Autodesk Inventor part; units mm, degrees
ref_plane "YZ Plane" through (0, 0, 0) normal (1, 0, 0) x (0, 1, 0)
ref_plane "XZ Plane" through (0, 0, 0) normal (0, 1, 0) x (-1, 0, 0)
ref_plane "XY Plane" through (0, 0, 0) normal (0, 0, 1) x (1, 0, 0)
sketch "Sketch1" plane through (0, 0, 0) normal (1, 0, 0) x (0, 1, 0)
  arc A0 (-107.5189, 2.6268) -> (-107.5189, -2.6268) centre (-105.3147, 0) ccw construction
  line L0 (-105.5687, 3.175) -> (-105.5687, -3.175) construction
  line L1 (-107.5189, 2.6268) -> (-107.5189, 4.635) construction
  line L2 (-106.3625, 6.7721) -> (-106.3625, 3.5971) construction
  line L3 (-107.5189, 2.6268) -> (-106.3625, 3.5971) construction
  line L4 (-107.5189, -2.6268) -> (-106.3625, -3.5971) construction
  line L5 (-131.7625, 6.7721) -> (-131.7625, -6.7721) construction
  line L6 (-131.7625, 6.7721) -> (-106.3625, 6.7721) construction
  line L7 (-131.7625, -6.7721) -> (-106.3625, -6.7721) construction
  line L8 (-106.3625, -6.7721) -> (-106.3625, -3.5971) construction
  circle A1 centre (-105.5687, 0) radius 3.175 construction
  line L9 (-35.1032, 0) -> (87.3968, 0) construction
  line L10 (-104.775, 6.7721) -> (-104.775, 3.5971)
  line L11 (-104.775, -6.7721) -> (-104.775, -3.5971)
  line L12 (-103.6186, 2.6268) -> (-104.775, 3.5971)
  line L13 (-103.6186, -2.6268) -> (-104.775, -3.5971)
  arc A2 (-103.6186, -2.6268) -> (-103.6186, 2.6268) centre (-105.8227, 0) ccw
  line L14 (-79.375, 6.7721) -> (-79.375, -6.7721)
  line L15 (0, -7.2584) -> (0, 7.2584) construction
  line L16 (-79.375, -6.7721) -> (-104.775, -6.7721)
  line L17 (-79.375, 6.7721) -> (-104.775, 6.7721) construction
  line L18 (-104.775, 6.7721) -> (-104.775, 17.0404)
  line L19 (-104.775, 17.0404) -> (-79.375, 17.0404)
  line L20 (-79.375, 17.0404) -> (-79.375, 6.7721)
  line L21 (-90.4875, 22.7342) -> (-90.4875, 17.0404) construction
  point P0 (0, 0)
  point P1 (0, 0)
  point P2 (-108.7437, 0)
  point P3 (-131.7625, 0)
  point P4 (-19.1031, 0)
  point P5 (0, 7.2584)
  point P6 (0, 0)
  point P7 (-143.7622, 15.4465)
  dimension "d0" = 6.35
  dimension "d1" = 3.429
  dimension "d2" = 50
  dimension "d3" = 3.175
  dimension "d4" = 1.5875
  dimension "d5" = 158.75
  dimension "d7" = 25.4
  dimension "d8" = 25.4
  dimension "d9" = 180.975
  dimension "d23" = 23.8125
revolve "Revolution1" add sketch "Sketch1" angle 360 about axis through (0, 0, -7.2584) along (0, 0, 1)
sketch "Sketch2" plane through (0, 0, 17.0404) normal (0, 0, 1) x (1, 0, 0)
  point P0 (0, 0)
  point P1 (0, -90.4875)
  point P2 (70.746, -56.418)
  point P3 (88.2188, 20.1354)
  point P4 (39.2611, 81.5264)
  point P5 (-39.2611, 81.5264)
  point P6 (-88.2188, 20.1354)
  point P7 (-70.746, -56.418)
  dimension "d11" = 90.4875
  dimension "d14" = 360
hole "Hole1" at (0, -90.4875, 17.0404) at (70.746, -56.418, 17.0404) at (88.2188, 20.1354, 17.0404) at (39.2611, 81.5264, 17.0404) at (-39.2611, 81.5264, 17.0404) at (-88.2188, 20.1354, 17.0404) at (-70.746, -56.418, 17.0404) direction (0, 0, -1) diameter 6.12 depth 7.9375 tip angle 118
equation "\"d8\" = d7"
properties part number "3DPRINT,TURRET,BEARING,INNER" material "Nylon 6/6"
Can you work these out from the model? Positions are in its coordinate system, mm. A direction names the side the tool comes from. Round coordinates to 2 decimals unless told otherwise and drop trailing zeros. Loops run counter-clockwise (first coordinate to the right, second up) from the corner with the lowest first, then second, coordinate; pieces in that order, holes last.
Item 1: Please list where these lines run through material, in increasing order: L1, parallel to X at y = -1, z = -4.5; L2, parallel to Y at x = -49, z = -4.5; L3, parallel to X at y = 7, z = 7.
Item 2: Which directions (+Z, -Z, +X, -X, +Y, -Y) give clear straight access to the entire face, cutting with the end or side of a thin tool? Please do faces 1 (the cylindrical face through (-102.283, 22.713, -5.162)), 2 (the cylindrical face through (90.93, 18.72, 13.02)).
Item 3: If we mould it in two halves opening along X, with no side actions, what happens to faces 3 (the flat face through (78, 16, -6.772)), 4 (the cylindrical face through (102.283, 22.713, 10.225)), 5 (the cylindrical face through (-73.78, -56.02, 13.02))? For each: +X half, -X half, draft (parallel to the pull), parting line (faces both ways), or undercut.
Item 4: Will these pins go through, and if not, where does the flat tip stop? pin 1 Ø2 at (y, z) = (-49.5, 6.5) entering from +X; pin 2 Ø7 at (x, y) = (-70.746, -56.418) entering from +Z; pin 3 Ø1 at (x, z) = (23, 1) entering from -Y; pin 4 Ø1 at (x, z) = (-16.5, 12.5) entering from -Y.
Item 5: Suppose I cut it at A-A, the plane y = 0. Write out the boundary of the cut face in (x, z) (3 decimals).
Reported:
1. L1: x = -104.77 to -79.37, 79.37 to 104.77
1. L2: y = -92.61 to -62.45, 62.45 to 92.61
1. L3: x = -104.54 to -79.07, 79.07 to 104.54
2. face 1: +Z, -Z
2. face 2: +Z
3. face 3: draft
3. face 4: parting line
3. face 5: undercut
4. pin 1: stops at x = 92.87
4. pin 2: stops at z = 17.04
4. pin 3: stops at y = -100.16
4. pin 4: stops at y = -103.55
5. outline: (-104.775, -6.772) - (-79.375, -6.772) - (-79.375, 17.04) - (-104.775, 17.04) - (-104.775, 3.597) - (-103.619, 2.627) arc R3.429 cw to (-103.619, -2.627) - (-104.775, -3.597) - close; (79.375, -6.772) - (104.775, -6.772) - (104.775, -3.597) - (103.619, -2.627) arc R3.429 cw to (103.619, 2.627) - (104.775, 3.597) - (104.775, 17.04) - (79.375, 17.04) - close
